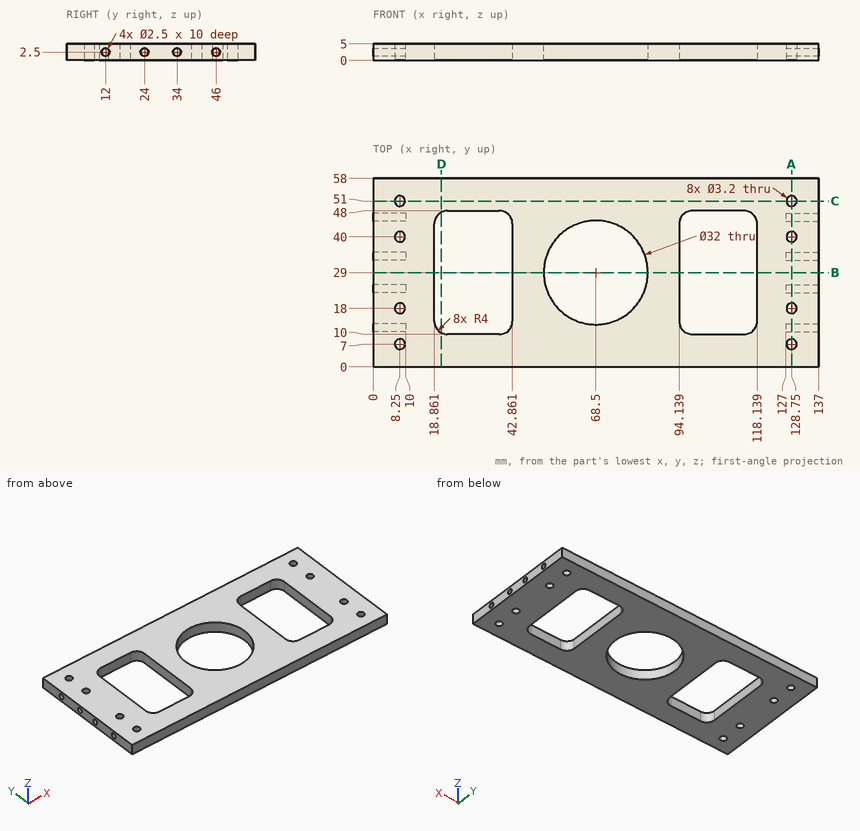
Print and shaded views of the part. All mm, measured from the part's lowest x, y and z. Give positions to 0.01 mm unless a question says otherwise; leave off trailing zeros. Loops run counter-clockwise (first coordinate to the right, second up) from the corner with the lowest first, then second, coordinate; pieces in that order, holes last. Notation, with made-up numbers: (-35.5, 86) - (4.5, 86) arc R14 ccw to (4.5, 91) - close; hole circle Ø5 at (-14.75, 3.25). An arc over 180 degrees is marked (long way). One line per item, written item: value. Start each with the question number.
1. Probe L1, parallel to Y at x = 2.75, z = 2.5; L2, parallel to Y at x = 108, z = 0.2; L3, parallel to X at y = 25, z = 2. List the from-to ranges inside material, lowest first. Write a range as from..to.
2. Pin check, flat tip, straight feed: pin 1 (1.5 mm diameter, centred on x = 36, z = 2, fed in from -Y). Stop position of the tip, or through.
3. Slice it at A-A (x = 128.75). Give the number of separate pieces and of enclosed holes in the cut face, plus the area to 3 significant figures.
4. Slice it at C-C (y = 51). List the corners of the cut face in (x, z), plus the area to 3 significant figures.
5. Slice it at D-D (x = 21). List the corners of the cut face in (y, z).
6. Slice it at B-B (y = 29). List the corners of the cut face in (x, z), plus the area to 3 significant figures.
Solution:
1. L1: y = 0..10.75, 13.25..22.75, 25.25..32.75, 35.25..44.75, 47.25..58
1. L2: y = 0..10, 48..58
1. L3: x = 10..18.86, 42.86..53.01, 83.99..94.14, 118.14..127
2. pin 1: stops at y = 0
3. separate pieces: 5
3. enclosed holes: 4
3. area: 206 mm^2
4. outline: (0, 0) - (6.65, 0) - (6.65, 5) - (0, 5) - close; (9.85, 0) - (127.15, 0) - (127.15, 5) - (9.85, 5) - close; (130.35, 0) - (137, 0) - (137, 5) - (130.35, 5) - close
4. area: 653 mm^2
5. outline: (0, 0) - (10.46, 0) - (10.46, 5) - (0, 5) - close; (47.54, 0) - (58, 0) - (58, 5) - (47.54, 5) - close
6. outline: (0, 0) - (18.86, 0) - (18.86, 5) - (0, 5) - close; (42.86, 0) - (52.5, 0) - (52.5, 5) - (42.86, 5) - close; (84.5, 0) - (94.14, 0) - (94.14, 5) - (84.5, 5) - close; (118.14, 0) - (137, 0) - (137, 5) - (118.14, 5) - close
6. area: 285 mm^2
